```python
from build123d import *

# Parameters (mm, degrees)
BOSS_EXTRUDE2_DEPTH = 25
CIRPATTERN2_COUNT   = 4
CUT_EXTRUDE2_DEPTH  = 2.5
FILLET1_R           = 10
SKETCH8_R           = 1.7
CUT_EXTRUDE3_DEPTH  = 128.671453348
CIRPATTERN3_COUNT   = 4
SKETCH10_W          = 4
SKETCH10_H          = 2
CUT_EXTRUDE4_DEPTH  = 128.671453348
SKETCH11_W          = 8
SKETCH11_H          = 10
CUT_EXTRUDE5_DEPTH  = 7
CIRPATTERN4_COUNT   = 4


with BuildPart() as part:
    # Sketch2 → Boss-Extrude2 (new, symmetric)
    with BuildSketch(Plane.XY):
        Polygon((-50, 0), (50, 0), (50, 5), (90, 5), (90, 10), (-90, 10), (-90, 5), (-50, 5), align=None)
    boss_extrude2 = extrude(amount=BOSS_EXTRUDE2_DEPTH, both=True)

    # CirPattern2: Boss-Extrude2 ×4 about axis
    cirpattern2_axis = Axis((0, 0, 0), (0, 1, 0))
    for i in range(1, CIRPATTERN2_COUNT):
        add(boss_extrude2.rotate(cirpattern2_axis, i * 360 / CIRPATTERN2_COUNT))

    # Sketch4 → Cut-Extrude2 (cut, symmetric)
    with BuildSketch(Plane(origin=(0, 10, 0), x_dir=(1, 0, 0), z_dir=(0, 1, 0))):
        Polygon((-3.5, 21.1), (-21.1, 21.1), (-21.1, -21.1), (21.1, -21.1), (21.1, 21.1), (3.5, 21.1), (3.5, 28.1), (-3.5, 28.1), align=None)
    extrude(amount=CUT_EXTRUDE2_DEPTH, both=True, mode=Mode.SUBTRACT)

    # Fillet1
    fillet1_edges = [part.edges().sort_by_distance(p)[0] for p in [
        (-25, 5, 25),
        (25, 5, -25),
        (25, 5, 25),
        (-25, 5, -25),
    ]]
    fillet(fillet1_edges, radius=FILLET1_R)

    # Sketch8 → Cut-Extrude3 (cut, through all)
    with BuildSketch(Plane(origin=(0, 10, 0), x_dir=(1, 0, 0), z_dir=(0, 1, 0))):
        with Locations(Location((-72.5, 0, 0), (0, 0, 270))):
            Circle(SKETCH8_R)
    cut_extrude3 = extrude(amount=-CUT_EXTRUDE3_DEPTH, mode=Mode.SUBTRACT)

    # CirPattern3: Cut-Extrude3 ×4 about axis
    cirpattern3_axis = Axis((0, 0, 0), (0, 1, 0))
    for i in range(1, CIRPATTERN3_COUNT):
        add(cut_extrude3.rotate(cirpattern3_axis, i * 360 / CIRPATTERN3_COUNT), mode=Mode.SUBTRACT)

    # Sketch10 → Cut-Extrude4 (cut, through all)
    with BuildSketch(Plane(origin=(0, 10, 0), x_dir=(1, 0, 0), z_dir=(0, 1, 0))):
        with Locations((-43.840620434, 2.5)):
            Rectangle(SKETCH10_W, SKETCH10_H)
        with Locations((-43.840620434, -2.5)):
            Rectangle(SKETCH10_W, SKETCH10_H)
    cut_extrude4 = extrude(amount=-CUT_EXTRUDE4_DEPTH, mode=Mode.SUBTRACT)

    # Sketch11 → Cut-Extrude5 (cut)
    with BuildSketch(Plane.XZ):
        with Locations((-43.840620434, 0)):
            Rectangle(SKETCH11_W, SKETCH11_H)
    cut_extrude5 = extrude(amount=-CUT_EXTRUDE5_DEPTH, mode=Mode.SUBTRACT)

    # CirPattern4: Cut-Extrude4, Cut-Extrude5 ×4 about axis
    cirpattern4_axis = Axis((0, 0, 0), (0, 1, 0))
    add([cut_extrude4.rotate(cirpattern4_axis, i * 360 / CIRPATTERN4_COUNT) for i in range(1, CIRPATTERN4_COUNT)], mode=Mode.SUBTRACT)
    add([cut_extrude5.rotate(cirpattern4_axis, i * 360 / CIRPATTERN4_COUNT) for i in range(1, CIRPATTERN4_COUNT)], mode=Mode.SUBTRACT)


solid = part.part
```
Work out the finished part from the listing and answer in its coordinate system (mm). A direction names the side the tool comes from. Coordinates: 2 decimals unless noted, no trailing zeros. Loops run counter-clockwise (first coordinate to the right, second up) from the corner with the lowest first, then second, coordinate; pieces in that order, holes last.
1) Section C-C (x = 56.5) is taken. Give the vertices of the cut face in (y, z), plus the area to 3 significant figures.
Results:
outline: (5, -25) - (10, -25) - (10, 25) - (5, 25) - close
area: 250 mm2
2) For faces 4 (the flat face through (-25, 6, -56)), 5 (the flat face through (25, 6, 57)), 6 (the flat face through (-25, 6, 57)), 7 (the flat face through (44, 7, 0)), determine the directions among +Z, -Z, +X, -X, +Y, -Y from which every point of the face is accessible in a straight line to the end or side of a thin tool.
Results:
face 4: -Z, -X, +Y, -Y
face 5: +Z, +X, +Y, -Y
face 6: +Z, -X, +Y, -Y
face 7: -Y
3) Section A-A (y = 3) is taken. Give the number of separate pieces and of enclosed holes in the cut face, plus the area to 3 significant figures.
Results:
separate pieces: 1
enclosed holes: 4
area: 7,270 mm2
4) Consider probe 1 along Z at (x, y) = (0, 7.6); probe 2 along X at (y, z) = (6.4, 0); probe 3 along Z at (x, y) = (-72.5, 8.3). Determine where each line is inside the solid, lowest interval first.
Results:
probe 1: z = -90 to -74.2, -70.8 to -28.1, 21.1 to 70.8, 74.2 to 90
probe 2: x = -90 to -74.2, -70.8 to -47.84, -39.84 to 39.84, 47.84 to 70.8, 74.2 to 90
probe 3: z = -25 to -1.7, 1.7 to 25
5) Flat-ended cylindrical pins translate along their axes: pin 1 (0.9 mm diameter, centred on y = 8, z = -43.5, fed in from -X); pin 2 (5 mm diameter, centred on x = 62, y = 6, fed in from -Z); pin 3 (4 mm diameter, centred on y = 3.5, z = 24.5, fed in from -X); pin 4 (12 mm diameter, centred on x = 61, z = -7, fed in from -Y). Find the tip coordinate at first contact, or state that the pin passes through.
Results:
pin 1: stops at x = -25
pin 2: stops at z = -25
pin 3: stops at x = -90
pin 4: stops at y = 5
6) Section D-D (z = 59.5) is taken. Give the vertices of the cut face in (x, y), plus the area to 3 significant figures.
Results:
outline: (-25, 5) - (25, 5) - (25, 10) - (-25, 10) - close
area: 250 mm2
7) Section B-B (z = 19) is taken. Give the vertices of the cut face in (x, y), plus the area to 3 significant figures.
Results:
outline: (-90, 5) - (-50, 5) - (-50, 0) - (50, 0) - (50, 5) - (90, 5) - (90, 10) - (21.1, 10) - (21.1, 7.5) - (-21.1, 7.5) - (-21.1, 10) - (-90, 10) - close
area: 1,290 mm2
8) For a pull along Z with two mould halves and no side action, classify faces 1 (the flat face through (70, 5, 0)), 2 (the flat face through (-5, 3, -44)), 3 (the flat face through (0, 3, 50)) as +Z half, -Z half, draft (parallel to the pull), parting line (faces both ways), or undercut.
Results:
face 1: draft
face 2: undercut
face 3: +Z half
